Could you check a few things on this drawing? It's one solid part, dimensions in mm from its lowest x, y, z. A direction names the side the tool comes from. Coordinates: 2 decimals unless noted, no trailing zeros. Loops run counter-clockwise (first coordinate to the right, second up) from the corner with the lowest first, then second, coordinate; pieces in that order, holes last. Notation, with made-up numbers: M 77.25,-25 L 82.25,-25 A26 ccw 82.25,13 Z; hole C 38,-24 d6. An arc over 180 degrees is marked long. Use one line per item in the form item = value. Start each with the question number.
(1) Imagine slicing it at C-C, the plane y = 93.5. Please give me the cut outline in (x, z), and give its area (3 significant figures).
(2) Imagine slicing it at A-A, the plane z = 20. Please give me the cut outline in (x, y), and give its area (3 significant figures).
(3) Please list where these lines run through material, in increasing order: L1, parallel to X at y = 67, z = 9.5; L2, parallel to X at y = 53, z = 3.
(4) Thinking about a two-plate mould opening in Y: for the marked faces 1, 2 and 3, which applies, +Y half, -Y half, draft (parallel to the pull), parting line (faces both ways), or undercut?
(5) Will these pins go through, and if not, where does the flat tip stop? P1, Ø9, axis at y = 59.5, z = 17.5, coming from the -X side; P2, Ø8, axis at x = 39, y = 53.5, coming from the +Z side; P3, Ø1.5, axis at x = 50.5, y = 95.5, coming from the +Z side.
(6) On a 3-axis mill with a long thin cutter (end or side, diameter ignored), from which of +Z, -Z, +X, -X, +Y, -Y can I reach the whole of each face in a straight line? I mean the marked faces 4 and 5. Say none if no direction works.
(7) Imagine slicing it at B-B, the plane x = 53.34. Please give me the cut outline in (y, z), and give its area (3 significant figures).
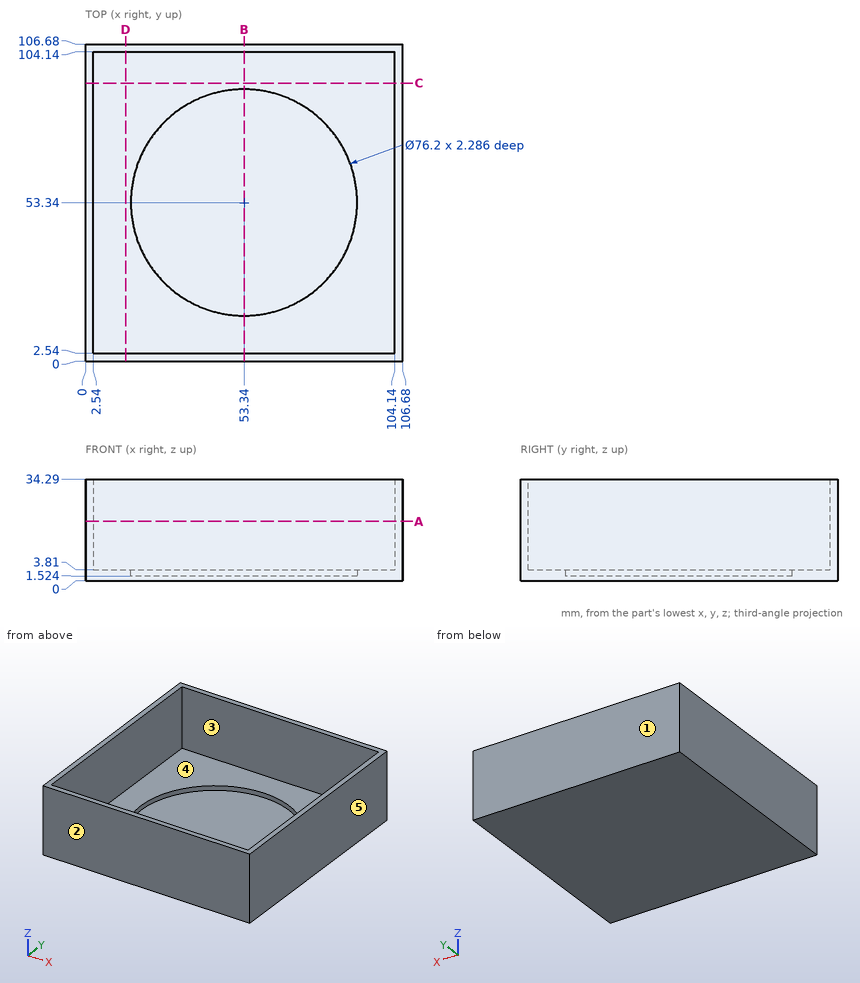
Answer:
q1.outline = M 0,0 L 106.68,0 L 106.68,34.29 L 104.14,34.29 L 104.14,3.81 L 2.54,3.81 L 2.54,34.29 L 0,34.29 Z
q1.area = 561 mm²
q2.outline = M 0,0 L 106.68,0 L 106.68,106.68 L 0,106.68 Z; hole M 2.54,2.54 L 104.14,2.54 L 104.14,104.14 L 2.54,104.14 Z
q2.area = 1,060 mm²
q3.L1 = 0 to 2.54, 104.14 to 106.68
q3.L2 = 0 to 15.24, 91.44 to 106.68
q4.face_1 = +Y half
q4.face_2 = -Y half
q4.face_3 = undercut
q5.P1 = 0
q5.P2 = 1.52
q5.P3 = 3.81
q6.face_4 = +Z
q6.face_5 = +Z, -Z, +X, +Y, -Y
q7.outline = M 0,0 L 106.68,0 L 106.68,34.29 L 104.14,34.29 L 104.14,3.81 L 91.44,3.81 L 91.44,1.52 L 15.24,1.52 L 15.24,3.81 L 2.54,3.81 L 2.54,34.29 L 0,34.29 Z
q7.area = 387 mm²
